Can you work these out from the drawing? Everything is in mm from the part's minimum corner. A direction names the side the tool comes from. Give positions to 0.01 mm unless a question says otherwise; leave off trailing zeros. Write each loop counter-clockwise with the first axis right and the second up, starting at its lowest first coordinate (ties: lowest second). Pieces come first, ordered by that corner, then holes. Notation, with made-up numbers: (-7, -39) - (34, -39) arc R29 ccw to (34, -18) - close; hole circle Ø1 at (27.5, 5.5). An arc over 180 degrees is marked (long way). Use a Markdown table: item, result.
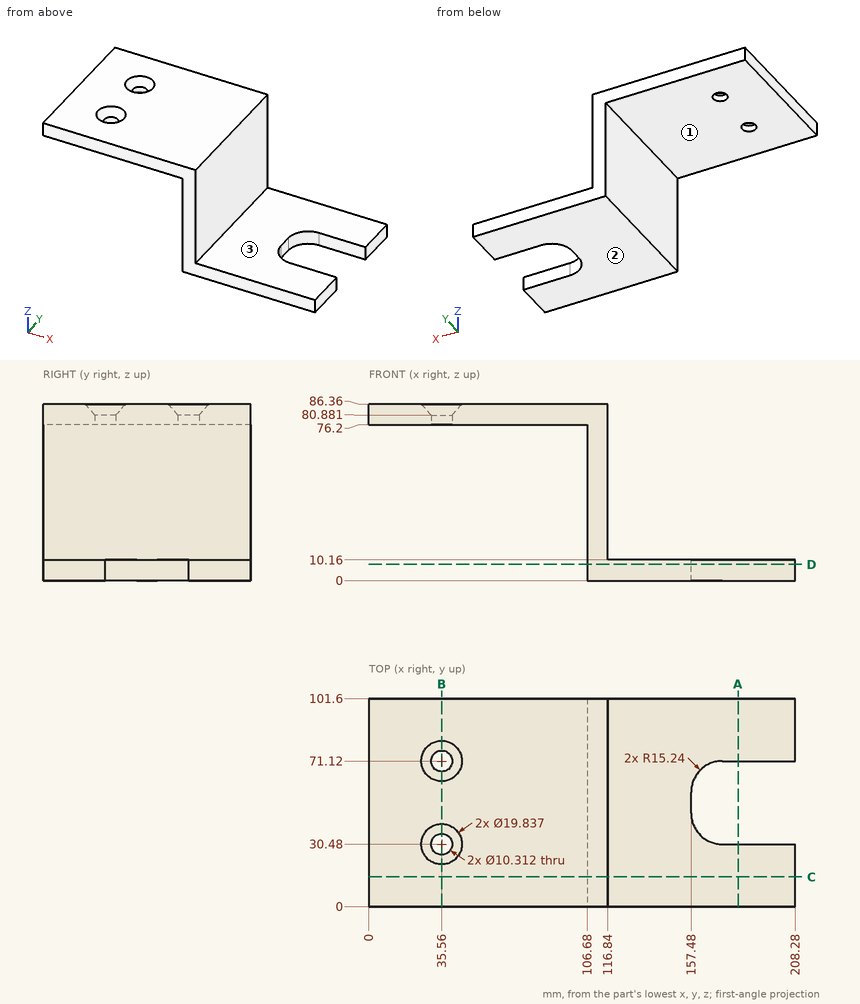
Item 1: If we section it at A-A, the plane x = 180.5: Write out the boundary of the cut face in (y, z), plus the area to 3 significant figures.
Values:
| item | result |
|---|---|
| outline | (0, 0) - (30.48, 0) - (30.48, 10.16) - (0, 10.16) - close; (71.12, 0) - (101.6, 0) - (101.6, 10.16) - (71.12, 10.16) - close |
| area | 619 mm2 |
Item 2: Will these pins go through, and if not, where does the flat tip stop? pin 1 Ø12 at (y, z) = (72, 72.5) entering from +X; pin 2 Ø8 at (y, z) = (75, 46) entering from -X; pin 3 Ø16.5 at (x, y) = (35.56, 71.12) entering from -Z; pin 4 Ø6 at (x, y) = (35.56, 30.48) entering from -Z.
Values:
| item | result |
|---|---|
| pin 1 | stops at x = 116.84 |
| pin 2 | stops at x = 106.68 |
| pin 3 | stops at z = 76.2 |
| pin 4 | passes through |
Item 3: If we section it at C-C, the plane y = 14.5: Write out the boundary of the cut face in (x, z), plus the area to 3 significant figures.
Values:
| item | result |
|---|---|
| outline | (0, 76.2) - (106.68, 76.2) - (106.68, 0) - (208.28, 0) - (208.28, 10.16) - (116.84, 10.16) - (116.84, 86.36) - (0, 86.36) - close |
| area | 2,890 mm2 |
Item 4: If we section it at B-B, the plane x = 35.56: Write out the boundary of the cut face in (y, z).
Values:
| item | result |
|---|---|
| outline | (0, 76.2) - (25.32, 76.2) - (25.32, 80.88) - (20.56, 86.36) - (0, 86.36) - close; (35.64, 76.2) - (65.96, 76.2) - (65.96, 80.88) - (61.2, 86.36) - (40.4, 86.36) - (35.64, 80.88) - close; (76.28, 76.2) - (101.6, 76.2) - (101.6, 86.36) - (81.04, 86.36) - (76.28, 80.88) - close |
Item 5: I need wall thicknesses on line 1 along Y through (x, z) = (35.56, 79.15); line 2 along Y through (x, z) = (35, 78) (1 decimal); line 3 along X through (y, z) = (30.48, 78.2). Which ranges of each line are inside material? Lowest first, please. Write a range as [from, to].
Values:
| item | result |
|---|---|
| line 1 | y = [0, 25.32], [35.64, 65.96], [76.28, 101.6] |
| line 2 | y = [0, 25.4], [35.6, 66], [76.2, 101.6] |
| line 3 | x = [0, 30.4], [40.72, 116.84] |
Item 6: If we section it at D-D, the plane z = 8: Write out the boundary of the cut face in (x, y), plus the area to 3 significant figures.
Values:
| item | result |
|---|---|
| outline | (106.68, 0) - (208.28, 0) - (208.28, 30.48) - (172.72, 30.48) arc R15.24 cw to (157.48, 45.72) - (157.48, 55.88) arc R15.24 cw to (172.72, 71.12) - (208.28, 71.12) - (208.28, 101.6) - (106.68, 101.6) - close |
| area | 8,360 mm2 |
Item 7: For the marked faces 1, 2 and 3, which set-ups out of +Z, -Z, +X, -X, +Y, -Y let a thin tool reach every point of the face, with its end or its side?
Values:
| item | result |
|---|---|
| face 1 | -Z, -X, +Y, -Y |
| face 2 | -Z, +X, -X, +Y, -Y |
| face 3 | +Z, +X, +Y, -Y |
